from build123d import *

# Parameters (mm, degrees)
SKETCH1_R           = 7.493
BOSS_EXTRUDE1_DEPTH = 0.8128


with BuildPart() as part:
    # Sketch1 → Boss-Extrude1 (new body)
    with BuildSketch(Plane.XY):
        with BuildLine():
            Line((-6.457079781, 35.480882848), (-3.305892697, 41.587736724))
            Line((-3.305892697, 41.587736724), (2.330830076, 41.587736724))
            Line((2.330830076, 41.587736724), (1.007052256, 37.443040758))
            ThreePointArc((1.007052256, 37.443040758), (1.307937447, 35.269279401), (3.190317281, 34.141264998))
            ThreePointArc((3.190317281, 34.141264998), (3.482262993, 34.112724084), (3.773953868, 34.081686757))
            ThreePointArc((3.773953868, 34.081686757), (5.813520367, 34.271336714), (7.612382182, 35.251078913))
            Line((7.612382182, 35.251078913), (12.860691234, 39.687169127))
            Line((12.860691234, 39.687169127), (18.068344035, 37.530088709))
            Line((18.068344035, 37.530088709), (15.259226323, 34.207476777))
            ThreePointArc((15.259226323, 34.207476777), (14.705345535, 32.084039374), (16.012765313, 30.321534378))
            ThreePointArc((16.012765313, 30.321534378), (16.271565846, 30.183443225), (16.529175604, 30.043143208))
            ThreePointArc((16.529175604, 30.043143208), (18.486065244, 29.437848614), (20.522927965, 29.654617765))
            Line((20.522927965, 29.654617765), (27.069351508, 31.744589796))
            Line((27.069351508, 31.744589796), (31.055116405, 27.758824899))
            Line((31.055116405, 27.758824899), (27.188321507, 25.764134549))
            ThreePointArc((27.188321507, 25.764134549), (25.86399807, 24.014295194), (26.397414982, 21.885625015))
            ThreePointArc((26.397414982, 21.885625015), (26.583670301, 21.659006749), (26.767980192, 21.430803448))
            ThreePointArc((26.767980192, 21.430803448), (28.344274264, 20.122714917), (30.309044005, 19.543509881))
            Line((30.309044005, 19.543509881), (37.156948399, 18.969184434))
            Line((37.156948399, 18.969184434), (39.314028817, 13.761531633))
            Line((39.314028817, 13.761531633), (34.978241205, 13.398436388))
            ThreePointArc((34.978241205, 13.398436388), (33.085091357, 12.288592261), (32.763297513, 10.117827636))
            ThreePointArc((32.763297513, 10.117827636), (32.848651934, 9.837182834), (32.931602448, 9.555818134))
            ThreePointArc((32.931602448, 9.555818134), (33.88732447, 7.744080287), (35.480882848, 6.457079781))
            Line((35.480882848, 6.457079781), (41.587736724, 3.305892697))
            Line((41.587736724, 3.305892697), (41.587736724, -2.330830076))
            Line((41.587736724, -2.330830076), (37.443040758, -1.007052256))
            ThreePointArc((37.443040758, -1.007052256), (35.269279401, -1.307937447), (34.141264998, -3.190317281))
            ThreePointArc((34.141264998, -3.190317281), (34.112724084, -3.482262993), (34.081686757, -3.773953868))
            ThreePointArc((34.081686757, -3.773953868), (34.271336714, -5.813520367), (35.251078913, -7.612382182))
            Line((35.251078913, -7.612382182), (39.687169127, -12.860691234))
            Line((39.687169127, -12.860691234), (37.530088709, -18.068344035))
            Line((37.530088709, -18.068344035), (34.207476777, -15.259226323))
            ThreePointArc((34.207476777, -15.259226323), (32.084039374, -14.705345535), (30.321534378, -16.012765313))
            ThreePointArc((30.321534378, -16.012765313), (30.183443225, -16.271565846), (30.043143208, -16.529175604))
            ThreePointArc((30.043143208, -16.529175604), (29.437848614, -18.486065244), (29.654617765, -20.522927965))
            Line((29.654617765, -20.522927965), (31.744589796, -27.069351508))
            Line((31.744589796, -27.069351508), (27.758824899, -31.055116405))
            Line((27.758824899, -31.055116405), (25.764134549, -27.188321507))
            ThreePointArc((25.764134549, -27.188321507), (24.014295194, -25.86399807), (21.885625015, -26.397414982))
            ThreePointArc((21.885625015, -26.397414982), (21.659006749, -26.583670301), (21.430803448, -26.767980192))
            ThreePointArc((21.430803448, -26.767980192), (20.122714917, -28.344274264), (19.543509881, -30.309044005))
            Line((19.543509881, -30.309044005), (18.969184434, -37.156948399))
            Line((18.969184434, -37.156948399), (13.761531633, -39.314028817))
            Line((13.761531633, -39.314028817), (13.398436388, -34.978241205))
            ThreePointArc((13.398436388, -34.978241205), (12.288592261, -33.085091357), (10.117827636, -32.763297513))
            ThreePointArc((10.117827636, -32.763297513), (9.837182834, -32.848651934), (9.555818134, -32.931602448))
            ThreePointArc((9.555818134, -32.931602448), (7.744080287, -33.88732447), (6.457079781, -35.480882848))
            Line((6.457079781, -35.480882848), (3.305892697, -41.587736724))
            Line((3.305892697, -41.587736724), (-2.330830076, -41.587736724))
            Line((-2.330830076, -41.587736724), (-1.007052256, -37.443040758))
            ThreePointArc((-1.007052256, -37.443040758), (-1.307937447, -35.269279401), (-3.190317281, -34.141264998))
            ThreePointArc((-3.190317281, -34.141264998), (-3.482262993, -34.112724084), (-3.773953868, -34.081686757))
            ThreePointArc((-3.773953868, -34.081686757), (-5.813520367, -34.271336714), (-7.612382182, -35.251078913))
            Line((-7.612382182, -35.251078913), (-12.860691234, -39.687169127))
            Line((-12.860691234, -39.687169127), (-18.068344035, -37.530088709))
            Line((-18.068344035, -37.530088709), (-15.259226323, -34.207476777))
            ThreePointArc((-15.259226323, -34.207476777), (-14.705345535, -32.084039374), (-16.012765313, -30.321534378))
            ThreePointArc((-16.012765313, -30.321534378), (-16.271565846, -30.183443225), (-16.529175604, -30.043143208))
            ThreePointArc((-16.529175604, -30.043143208), (-18.486065244, -29.437848614), (-20.522927965, -29.654617765))
            Line((-20.522927965, -29.654617765), (-27.069351508, -31.744589796))
            Line((-27.069351508, -31.744589796), (-31.055116405, -27.758824899))
            Line((-31.055116405, -27.758824899), (-27.188321507, -25.764134549))
            ThreePointArc((-27.188321507, -25.764134549), (-25.86399807, -24.014295194), (-26.397414982, -21.885625015))
            ThreePointArc((-26.397414982, -21.885625015), (-26.583670301, -21.659006749), (-26.767980192, -21.430803448))
            ThreePointArc((-26.767980192, -21.430803448), (-28.344274264, -20.122714917), (-30.309044005, -19.543509881))
            Line((-30.309044005, -19.543509881), (-37.156948399, -18.969184434))
            Line((-37.156948399, -18.969184434), (-39.314028817, -13.761531633))
            Line((-39.314028817, -13.761531633), (-34.978241205, -13.398436388))
            ThreePointArc((-34.978241205, -13.398436388), (-33.085091357, -12.288592261), (-32.763297513, -10.117827636))
            ThreePointArc((-32.763297513, -10.117827636), (-32.848651934, -9.837182834), (-32.931602448, -9.555818134))
            ThreePointArc((-32.931602448, -9.555818134), (-33.88732447, -7.744080287), (-35.480882848, -6.457079781))
            Line((-35.480882848, -6.457079781), (-41.587736724, -3.305892697))
            Line((-41.587736724, -3.305892697), (-41.587736724, 2.330830076))
            Line((-41.587736724, 2.330830076), (-37.443040758, 1.007052256))
            ThreePointArc((-37.443040758, 1.007052256), (-35.269279401, 1.307937447), (-34.141264998, 3.190317281))
            ThreePointArc((-34.141264998, 3.190317281), (-34.112724084, 3.482262993), (-34.081686757, 3.773953868))
            ThreePointArc((-34.081686757, 3.773953868), (-34.271336714, 5.813520367), (-35.251078913, 7.612382182))
            Line((-35.251078913, 7.612382182), (-39.687169127, 12.860691234))
            Line((-39.687169127, 12.860691234), (-37.530088709, 18.068344035))
            Line((-37.530088709, 18.068344035), (-34.207476777, 15.259226323))
            ThreePointArc((-34.207476777, 15.259226323), (-32.084039374, 14.705345535), (-30.321534378, 16.012765313))
            ThreePointArc((-30.321534378, 16.012765313), (-30.183443225, 16.271565846), (-30.043143208, 16.529175604))
            ThreePointArc((-30.043143208, 16.529175604), (-29.437848614, 18.486065244), (-29.654617765, 20.522927965))
            Line((-29.654617765, 20.522927965), (-31.744589796, 27.069351508))
            Line((-31.744589796, 27.069351508), (-27.758824899, 31.055116405))
            Line((-27.758824899, 31.055116405), (-25.764134549, 27.188321507))
            ThreePointArc((-25.764134549, 27.188321507), (-24.014295194, 25.86399807), (-21.885625015, 26.397414982))
            ThreePointArc((-21.885625015, 26.397414982), (-21.659006749, 26.583670301), (-21.430803448, 26.767980192))
            ThreePointArc((-21.430803448, 26.767980192), (-20.122714917, 28.344274264), (-19.543509881, 30.309044005))
            Line((-19.543509881, 30.309044005), (-18.969184434, 37.156948399))
            Line((-18.969184434, 37.156948399), (-13.761531633, 39.314028817))
            Line((-13.761531633, 39.314028817), (-13.398436388, 34.978241205))
            ThreePointArc((-13.398436388, 34.978241205), (-12.288592261, 33.085091357), (-10.117827636, 32.763297513))
            ThreePointArc((-10.117827636, 32.763297513), (-9.837182834, 32.848651934), (-9.555818134, 32.931602448))
            ThreePointArc((-9.555818134, 32.931602448), (-7.744080287, 33.88732447), (-6.457079781, 35.480882848))
        make_face()
        Circle(SKETCH1_R, mode=Mode.SUBTRACT)
    extrude(amount=BOSS_EXTRUDE1_DEPTH)


solid = part.part
Geometry: final body of the model. Coordinates: model frame, mm. A direction names the side the tool comes from. Give positions to 0.01 mm unless a question says otherwise; leave off trailing zeros. Use CSV: the item, a comma, the result in double quotes.
1. Mould query, pull axis X, two halves, no side actions, for faces 1 (the face through (29.034, 29.78, 0.401)), 2 (the face through (20.136, -28.319, 0.401)), 3 (the face through (-28.319, -20.136, 0.401)). Classes: +X half, -X half, draft (parallel to the pull), parting line (faces both ways), or undercut.
Answers below:
face 1,"+X half"
face 2,"undercut"
face 3,"-X half"
2. Access query for faces 4 (the face through (35.3, -1.29, 0.4)), 5 (the face through (35.89, -16.68, 0.4)), 6 (the face through (-26.775, 29.149, 0.401)), 7 (the face through (28.319, 20.136, 0.401)), 8 (the face through (-16.68, -35.89, 0.4)). Directions: +Z, -Z, +X, -X, +Y, -Y. A direction counts if a zero-diameter tool reaches every point of the face in a straight line with its end or side. Return the directions, or none.
Answers below:
face 4,"+Z, -Z"
face 5,"+Z, -Z, -Y"
face 6,"+Z, -Z, +Y"
face 7,"+Z, -Z, +X"
face 8,"+Z, -Z, -X"
3. Material intervals for line 1 along Y through (x, z) = (0, 0.6); line 2 along Y through (x, z) = (-36, 0.6); line 3 along X through (y, z) = (36.5, 0.3), sorted ascending. Write a range as from..to.
Answers below:
line 1,"-41.59..-7.49, 7.49..41.59"
line 2,"-19.07..-13.48, -6.19..0.98, 8.5..16.77"
line 3,"-19.02..-13.53, -5.93..0.89, 9.09..17.2"
4. Contact query for a flat-ended pin moving along its axis: pin 1 (9 mm diameter, centred on x = 0, y = 0, fed in from +Z). Output: stop coordinate, or through.
Answers below:
pin 1,"through"
